For this review, take the finished solid that the model builds, in its own axes (mm). A direction names the side the tool comes from. Coordinates: 2 decimals unless noted, no trailing zeros. Write each loop counter-clockwise with the first axis right and the second up, starting at its lowest first coordinate (ties: lowest second). Pieces come first, ordered by that corner, then holes.
1) We need section A-A on y = -46. Write out the cut boundary in (x, z), then the cut area to 3 significant figures.
2) For faces 1 (the face through (-34, 0, 2.5)), 2 (the face through (-10, -18, 0)), 3 (the face through (0, 22, -2.5)), 4 (the face through (-41, 15, 0)), list the 3-axis set-ups (+Z, -Z, +X, -X, +Y, -Y) from which the entire face can be reached by the end or side of a thin tool; tool diameter is ignored.
3) We need section B-B on x = 22. Write out the cut boundary in (y, z), then the cut area to 3 significant figures.
4) Mouldability with a two-part tool opening along X and no side actions: class faces 5 (the face through (22, 0, 2.5)), 6 (the face through (15, -41, 0)), 7 (the face through (0, 34, 2.5)) as pulls with the +X half, pulls with the -X half, needs draft (parallel to the pull), parting line crosses it, or undercut.
5) We need section C-C on z = 0. Give the number of separate pieces and of enclosed holes in the cut face, then the cut area to 3 significant figures.
6) To check wall thickness, follow line 1 along Z through (x, y) = (1, 44); line 2 along X through (y, z) = (-8, -1); line 3 along Y through (x, z) = (-28.5, 0.5). State the ranges of each line that lie inside material, in increasing order.
7) Insertion check: P1, Ø6, axis at x = 15.36, y = 0, coming from the +Z side; P2, Ø1.5, axis at y = 33, z = -4, coming from the +X side; P3, Ø4.5, axis at x = 40.36, y = 0, coming from the +Z side; P4, Ø4, axis at y = 36.5, z = -1, coming from the -X side. Each pin has a flat end and moves straight along its axis. Give the tip position at first contact, or say it passes through.
from build123d import *

# Parameters (mm, degrees)
F0_W           = 45.71068
F0_H           = 20
F0_W_2         = 20
F0_H_2         = 45.71068
F1_DEPTH       = 5
F4_DEPTH       = 120
F6_DEPTH       = 5
F6_DEPTH_BACK  = 25
F7_W           = 30
F7_H           = 10
F8_DEPTH       = 5
F8_DEPTH_BACK  = 25
F9_W           = 30
F9_H           = 10
F10_DEPTH      = 5
F10_DEPTH_BACK = 25
F11_W          = 30
F11_H          = 10
F12_DEPTH      = 5
F12_DEPTH_BACK = 25
F13_R          = 2.5
F14_DEPTH      = 10
F15_DEPTH      = 116.7
F16_DEPTH      = 135


with BuildPart() as f1:
    # F0 (on Top) → F1 (new body, symmetric)
    with BuildSketch(Plane.XY):
        with Locations((32.85534, 0)):
            Rectangle(F0_W, F0_H)
        Rectangle(F0_W_2, F0_H)
        with Locations((0, 32.85534)):
            Rectangle(F0_W_2, F0_H_2)
        with Locations((-32.85534, 0)):
            Rectangle(F0_W, F0_H)
        with Locations((0, -32.85534)):
            Rectangle(F0_W_2, F0_H_2)
    extrude(amount=F1_DEPTH, both=True)

    # F2 (on face) → F4 (cut)
    with BuildSketch(Plane.XZ.offset(55.71068)):
        with BuildLine():
            Line((-2.5, -2.5), (2.5, -2.5))
            ThreePointArc((2.5, -2.5), (5, 0), (2.5, 2.5))
            Line((2.5, 2.5), (-2.5, 2.5))
            ThreePointArc((-2.5, 2.5), (-5, 0), (-2.5, -2.5))
        make_face()
    extrude(amount=-F4_DEPTH, mode=Mode.SUBTRACT)

    # F5 (on face) → F6 (join, two sides)
    with BuildSketch(Plane.YZ.offset(10)) as f6_sk:
        Polygon((-25.71068, 5), (-55.71068, 5), (-55.71068, 0), (-55.71068, -5), (-25.71068, -5), align=None)
    extrude(amount=F6_DEPTH)
    extrude(f6_sk.sketch, amount=-F6_DEPTH_BACK)

    # F7 (on face) → F8 (join, two sides)
    with BuildSketch(Plane(origin=(-10, 0, 0), x_dir=(0, -1, 0), z_dir=(-1, 0, 0))) as f8_sk:
        with Locations((-40.71068, 0)):
            Rectangle(F7_W, F7_H)
    extrude(amount=F8_DEPTH)
    extrude(f8_sk.sketch, amount=-F8_DEPTH_BACK)

    # F9 (on face) → F10 (join, two sides)
    with BuildSketch(Plane(origin=(0, 10, 0), x_dir=(-1, 0, 0), z_dir=(0, 1, 0))) as f10_sk:
        with Locations((-40.71068, 0)):
            Rectangle(F9_W, F9_H)
    extrude(amount=F10_DEPTH)
    extrude(f10_sk.sketch, amount=-F10_DEPTH_BACK)

    # F11 (on face) → F12 (join, two sides)
    with BuildSketch(Plane(origin=(0, 10, 0), x_dir=(-1, 0, 0), z_dir=(0, 1, 0))) as f12_sk:
        with Locations((40.71068, 0)):
            Rectangle(F11_W, F11_H)
    extrude(amount=F12_DEPTH)
    extrude(f12_sk.sketch, amount=-F12_DEPTH_BACK)

    # F13 (on face) → F14 (cut)
    with BuildSketch(Plane.XY.offset(5)):
        with Locations((-27.85534, 0)):
            Circle(F13_R)
        with Locations((-15, 0)):
            Circle(F13_R)
        with Locations((-40.71068, 0)):
            Circle(F13_R)
        with Locations((27.85534, 0)):
            Circle(F13_R)
        with Locations((40.35534, 0)):
            Circle(F13_R)
        with Locations((15.35534, 0)):
            Circle(F13_R)
        with Locations((0, 27.85534)):
            Circle(F13_R)
        with Locations((0, 40.35534)):
            Circle(F13_R)
        with Locations((0, 15.35534)):
            Circle(F13_R)
        with Locations((0, -27.85534)):
            Circle(F13_R)
        with Locations((0, -15.35534)):
            Circle(F13_R)
        with Locations((0, -40.35534)):
            Circle(F13_R)
    extrude(amount=-F14_DEPTH, mode=Mode.SUBTRACT)

    # F2 (on face) → F15 (cut)
    with BuildSketch(Plane.XZ.offset(55.71068)):
        with BuildLine():
            Line((-2.5, -2.5), (2.5, -2.5))
            ThreePointArc((2.5, -2.5), (5, 0), (2.5, 2.5))
            Line((2.5, 2.5), (-2.5, 2.5))
            ThreePointArc((-2.5, 2.5), (-5, 0), (-2.5, -2.5))
        make_face()
    extrude(amount=-F15_DEPTH, mode=Mode.SUBTRACT)

    # F3 (on face) → F16 (cut)
    with BuildSketch(Plane.YZ.offset(55.71068)):
        with BuildLine():
            Line((-2.5, -2.5), (2.5, -2.5))
            ThreePointArc((2.5, -2.5), (5, 0), (2.5, 2.5))
            Line((2.5, 2.5), (-2.5, 2.5))
            ThreePointArc((-2.5, 2.5), (-5, 0), (-2.5, -2.5))
        make_face()
    extrude(amount=-F16_DEPTH, mode=Mode.SUBTRACT)


solid = f1.part
Result:
1. outline: (-15, -5) - (15, -5) - (15, 5) - (-15, 5) - close; hole (-2.5, -2.5) - (2.5, -2.5) arc R2.5 ccw to (2.5, 2.5) - (-2.5, 2.5) arc R2.5 ccw to start
1. area: 255 mm2
2. face 1: +X, -X
2. face 2: +Z, -Z
2. face 3: +Y, -Y
2. face 4: +Z, -Z, -X, +Y
3. outline: (-10, -5) - (10, -5) - (10, 5) - (-10, 5) - close; hole (-2.5, -2.5) - (2.5, -2.5) arc R2.5 ccw to (2.5, 2.5) - (-2.5, 2.5) arc R2.5 ccw to start
3. area: 155 mm2
4. face 5: needs draft
4. face 6: pulls with the +X half
4. face 7: undercut
5. separate pieces: 4
5. enclosed holes: 0
5. area: 3,130 mm2
6. line 1: z = -5 to -2.5, 2.5 to 5
6. line 2: x = -55.71 to -4.79, 4.79 to 55.71
6. line 3: y = -15 to -4.95, 4.95 to 15
7. P1: stops at z = 5
7. P2: stops at x = 15
7. P3: passes through
7. P4: stops at x = -15
